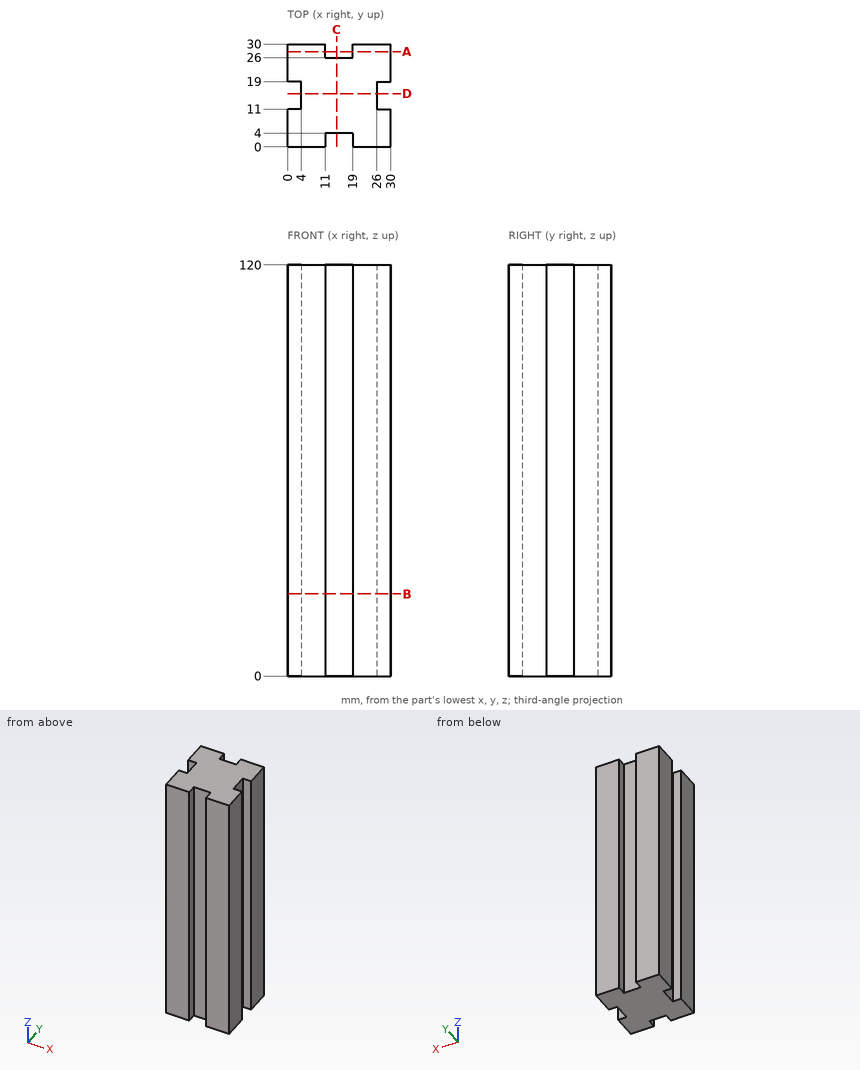
Check sheet for the drawn part. Datum: minimum x, y, z corner. Units: mm. Give positions to 0.01 mm unless a question says otherwise; leave off trailing zeros. Order: outer loops, then holes, each group sorted by start corner. A loop starts at its lowest first (then second) coordinate and runs counter-clockwise, first axis right, second up. Notation, with made-up numbers: (79, 4) -> (93, 4) arc R20 cw to (93, 24) -> close; hole circle Ø10 at (8, -1). An arc over 180 degrees is marked (long way). Use a Markdown table: item, result.
1) Section check C-C, the plane x = 14.25. Record the boundary of the cut face in (y, z).
Results:
| item | result |
|---|---|
| outline | (4, 0) -> (26, 0) -> (26, 120) -> (4, 120) -> close |
2) Depth check by flat-ended pin: pin 1 Ø1.5 at (y, z) = (12.5, 62) entering from -X; pin 2 Ø2.5 at (x, z) = (13.5, 74) entering from +Y. Enter the tip coordinate at first touch or a pass-through.
Results:
| item | result |
|---|---|
| pin 1 | x = 4 |
| pin 2 | y = 26 |
3) Section check B-B, the plane z = 24. Record the boundary of the cut face in (x, y), then the cut area to 3 significant figures.
Results:
| item | result |
|---|---|
| outline | (0, 0) -> (11, 0) -> (11, 4) -> (19, 4) -> (19, 0) -> (30, 0) -> (30, 11) -> (26, 11) -> (26, 19) -> (30, 19) -> (30, 30) -> (19, 30) -> (19, 26) -> (11, 26) -> (11, 30) -> (0, 30) -> (0, 19) -> (4, 19) -> (4, 11) -> (0, 11) -> close |
| area | 772 mm² |
4) Section check A-A, the plane y = 27.75. Record the boundary of the cut face in (x, z).
Results:
| item | result |
|---|---|
| outline | (0, 0) -> (11, 0) -> (11, 120) -> (0, 120) -> close; (19, 0) -> (30, 0) -> (30, 120) -> (19, 120) -> close |
5) Material ranges on probe 1 along Y at (x, z) = (3.75, 47); probe 2 along X at (y, z) = (11.75, 106.5), recorded low to high.
Results:
| item | result |
|---|---|
| probe 1 | 0 to 11, 19 to 30 |
| probe 2 | 4 to 26 |
